Source: CAD feature listing. Evaluate the final solid. Frame: model axes, mm. A direction names the side the tool comes from. Coordinates: 2 decimals unless noted, no trailing zeros. Order: outer loops, then holes, each group sorted by start corner. A loop starts at its lowest first (then second) coordinate and runs counter-clockwise, first axis right, second up.
Autodesk Inventor part; units mm, degrees
ref_plane "YZ Plane" through (0, 0, 0) normal (1, 0, 0) x (0, 1, 0)
ref_plane "XZ Plane" through (0, 0, 0) normal (0, 1, 0) x (-1, 0, 0)
ref_plane "XY Plane" through (0, 0, 0) normal (0, 0, 1) x (1, 0, 0)
ref_plane "작업 평면1" through (0, 0, 0) normal (0, 0, 1) x (1, 0, 0)
sketch "스케치1" plane through (0, 0, 0) normal (0, 0, 1) x (1, 0, 0)
  circle A0 centre (-7.7782, -7.7782) radius 1.55
  circle A1 centre (7.7782, -7.7782) radius 1.55
  circle A2 centre (7.7782, 7.7782) radius 1.55
  circle A3 centre (-7.7782, 7.7782) radius 1.55
  circle A4 centre (0, 0) radius 5
  circle A5 centre (0, 0) radius 13.9
  circle A6 centre (0, 11) radius 1.55
  circle A7 centre (11, 0) radius 1.55
  circle A8 centre (0, -11) radius 1.55
  circle A9 centre (-11, 0) radius 1.55
  circle A10 centre (11, 0) radius 1.35
  circle A11 centre (7.7782, 7.7782) radius 1.35
  circle A12 centre (0, 11) radius 1.35
  circle A13 centre (-7.7782, 7.7782) radius 1.35
  circle A14 centre (-11, 0) radius 1.35
  circle A15 centre (-7.7782, -7.7782) radius 1.35
  circle A16 centre (0, -11) radius 1.35
  circle A17 centre (7.7782, -7.7782) radius 1.35
  line L0 (13.9, 33.9052) -> (-13.9, 33.9052)
  line L1 (-3.1, 33.9052) -> (3.1, 33.9052)
  circle A18 centre (0, 0) radius 5.1
  circle A19 centre (0, 0) radius 13.9
  line L2 (-5.1, 0) -> (-5.1, -12.9306)
  line L3 (5.1, 0) -> (5.1, -12.9306)
  line L4 (13.9, 33.9052) -> (21, 33.9052)
  line L5 (21, 33.9052) -> (21, 13.9)
  line L6 (13.9, 13.9) -> (13.9, 13.9052)
  line L7 (-13.9, 33.9052) -> (-21, 33.9052)
  line L8 (-21, 33.9052) -> (-21, 13.9)
  line L9 (21, 13.9) -> (13.9, 0)
  line L10 (-21, 13.9) -> (-13.9, 0)
  line L11 (6.05, 33.9052) -> (-6.05, 33.9052)
  line L12 (-6.05, 33.9052) -> (-6.05, 27.8052)
  line L13 (-6.05, 27.8052) -> (6.05, 27.8052)
  line L14 (6.05, 27.8052) -> (6.05, 33.9052)
  circle A20 centre (10.6, 30.905) radius 1.35
  circle A21 centre (-10.6, 30.905) radius 1.35
  point P0 (13.9, 0)
  dimension "d1" = 2.7
  dimension "d4" = 360
  dimension "d34" = 0.1
  dimension "d37" = 12.1
  dimension "d38" = 6.1
  dimension "d44" = 2.7
  dimension "d45" = 2.7
extrude "돌출8" add sketch "스케치1" along normal blind 6 contours A0 | A1 | A2 | A3 | A5 L3 A18 L2 | A5 L10 L8 L7 L0 L12 L13 L14 L4 L5 L9 | A6 | A7 | A9 picked at (-7.5104, -2.4224)
fillet "모깎기2" radius 1 2 edges at (5.1, -12.9306, 3) (-5.1, -12.9306, 3)
sketch "스케치3" plane through (0, 0, 6) normal (0, 0, 1) x (1, 0, 0)
  line L0 (-6.05, 27.8052) -> (-6.05, 33.9052)
  line L1 (6.05, 27.8052) -> (-6.05, 27.8052)
  line L2 (6.05, 33.9052) -> (6.05, 27.8052)
  circle A0 centre (-6.05, 27.8052) radius 1
  circle A1 centre (6.05, 27.8052) radius 1
  point P0 (0, 0)
  dimension "d49" = 2
  dimension "d50" = 2
extrude "돌출9" cut sketch "스케치3" against normal blind 10
properties part number "leg_between" material "PMMA 플라스틱"
1. Section query D-D, the plane y = 11. Output: boundary loops of the cut face in (x, z).
2. Contact query for flat-ended pins moving along their axis: P1, Ø3, axis at x = 2, z = 4, coming from the +Y side; P2, Ø1.5, axis at x = -13.5, z = 2.5, coming from the -Y side; P3, Ø2, axis at x = 0, y = 11, coming from the -Z side. Output: stop coordinate, or through.
3. Material intervals for line 1 along X through (y, z) = (31, 4.8); line 2 along X through (y, z) = (-10, 1.25); line 3 along X through (y, z) = (-1, 3.15), sorted ascending.
4. Section query A-A, the plane x = 11. Output: boundary loops of the cut face in (y, z).
5. Section query B-B, the plane y = -2.5. Output: boundary loops of the cut face in (x, z), plus the area to 3 significant figures.
6. Section query C-C, the plane z = 2.75. Count the separate pieces of the cut face and the enclosed holes in it, plus the area to 3 significant figures.
7. Access query for faces 1 (the flat face through (5.1, -6, 3)), 2 (the flat face through (0, 27.805, 3)), 3 (the flat face through (0, 16, 0)). Directions: +Z, -Z, +X, -X, +Y, -Y. A direction counts if a zero-diameter tool reaches every point of the face in a straight line with its end or side. Return the directions, or none.
8. Draft query along X for faces 4 (the flat face through (0, 16, 6)), 5 (the flat face through (-5.1, -6, 3)), 6 (the flat face through (17.5, 7.05, 2.96)). Return one class per face: +X half, -X half, draft (parallel to the pull), parting line (faces both ways), or undercut.
Answer key:
1. outline: (-19.52, 0) - (-1.35, 0) - (-1.35, 6) - (-19.52, 6) - close; (1.35, 0) - (19.52, 0) - (19.52, 6) - (1.35, 6) - close
2. P1: stops at y = 27.81
2. P2: stops at y = -5.54
2. P3: passes through
3. line 1: x = -21 to -11.95, -9.25 to -6.05, 6.05 to 9.25, 11.95 to 21
3. line 2: x = -9.65 to -5.1, 5.1 to 9.65
3. line 3: x = -13.86 to -11.91, -10.09 to -5.1, 5.1 to 10.09, 11.91 to 13.86
4. outline: (-8.5, 0) - (-1.35, 0) - (-1.35, 6) - (-8.5, 6) - close; (1.35, 0) - (29.62, 0) - (29.62, 6) - (1.35, 6) - close; (32.19, 0) - (33.91, 0) - (33.91, 6) - (32.19, 6) - close
5. outline: (-13.67, 0) - (-5.1, 0) - (-5.1, 6) - (-13.67, 6) - close; (5.1, 0) - (13.67, 0) - (13.67, 6) - (5.1, 6) - close
5. area: 103 mm2
6. separate pieces: 1
6. enclosed holes: 9
6. area: 1,320 mm2
7. face 1: +Z, -Z, -Y
7. face 2: +Z, -Z, +Y
7. face 3: -Z, +X, -X, +Y, -Y
8. face 4: draft
8. face 5: undercut
8. face 6: +X half
